Design review of the part built by this model. Coordinates are the model's own, in mm. Face numbers are marked on the shaded views. Round coordinates to 2 decimals unless told otherwise and drop trailing zeros. Loops run counter-clockwise (first coordinate to the right, second up) from the corner with the lowest first, then second, coordinate; pieces in that order, holes last. Notation, with made-up numbers: M -16,43 L 5,43 A7 cw 5,50 Z; hole C 8,79.5 d5. An arc over 180 degrees is marked long. Use a Markdown table: item, result.
from build123d import *

# Parameters (mm, degrees)
F0_W     = 19.05
F0_H     = 19.05
F1_DEPTH = 76.2
F3_DEPTH = 25.4
F5_D     = 6.5278
F5_DEPTH = 12.7
F5_TIP   = 1.9611489744
F7_D     = 3.7973
F7_DEPTH = 12.7
F7_TIP   = 1.1408240143
F8_SIZE2 = 0.762
F8_SIZE  = 0.762


with BuildPart() as f1:
    # F0 (on Right) → F1 (new body)
    with BuildSketch(Plane.YZ):
        with Locations((-9.525, 9.525)):
            Rectangle(F0_W, F0_H)
    extrude(amount=F1_DEPTH)

    # F2 (on face) → F3 (cut)
    with BuildSketch(Plane.XZ.offset(19.05)):
        Polygon((50.8027122421, 0), (38.1, 12.7027122421), (38.1, 0), align=None)
        Polygon((38.1, 0), (38.1, 12.7027122421), (25.3972877579, 0), align=None)
    extrude(amount=-F3_DEPTH, mode=Mode.SUBTRACT)

    # F5
    with Locations(Plane.XY.offset(19.05)):
        with Locations((15.875, -9.525), (60.325, -9.525)):
            Hole(F5_D / 2, depth=F5_DEPTH)
            with Locations((0, 0, -(F5_DEPTH + F5_TIP / 2))):  # 118° drill point
                Cone(0, F5_D / 2, F5_TIP, mode=Mode.SUBTRACT)

    # F7
    with Locations(Plane(origin=(0, 0, 0), x_dir=(1, 0, 0), z_dir=(0, 0, -1))):
        with Locations((6.35, 9.525), (69.85, 9.525)):
            Hole(F7_D / 2, depth=F7_DEPTH)
            with Locations((0, 0, -(F7_DEPTH + F7_TIP / 2))):  # 118° drill point
                Cone(0, F7_D / 2, F7_TIP, mode=Mode.SUBTRACT)

    # F8
    f8_edges = [f1.edges().sort_by_distance(p)[0] for p in [
        (76.2, -19.05, 9.525),
        (76.2, 0, 9.525),
        (0, -19.05, 9.525),
        (0, 0, 9.525),
    ]]
    chamfer(f8_edges, length=F8_SIZE, length2=F8_SIZE2)


solid = f1.part
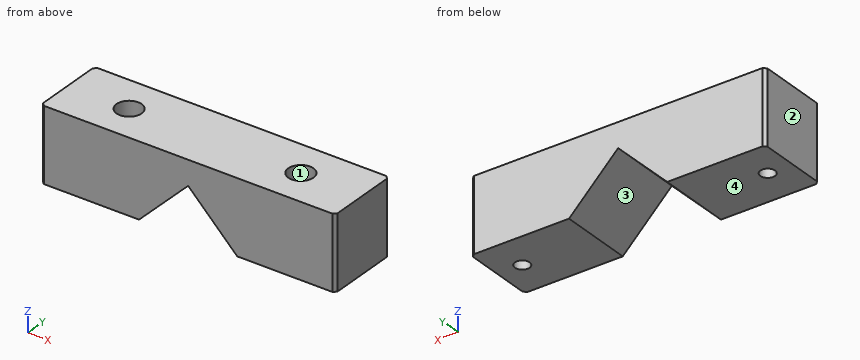
1. Wall thickness on line 1 along Y through (x, z) = (6.35, 6.75); line 2 along X through (y, z) = (-6.75, 12); line 3 along Y through (x, z) = (62, 11.25): over which ranges is each line inside the solid? List them lowest first. Write a range as from..to.
Check values:
| item | result |
|---|---|
| line 1 | y = -19.05..-11.42, -7.63..0 |
| line 2 | x = 0..14.16, 17.59..37.4, 38.8..58.61, 62.04..76.2 |
| line 3 | y = -19.05..-12.33, -6.72..0 |
2. Take a section at C-C on x = 41. Give the boundary of the cut face in (y, z).
Check values:
| item | result |
|---|---|
| outline | M -19.05,9.8 L 0,9.8 L 0,19.05 L -19.05,19.05 Z |
3. Insertion check: pin 1 (6 mm diameter, centred on x = 60.325, y = -9.525, fed in from +Z). The pin has a flat end and moves straight along its axis. Give the tip position at first contact, or say it passes through.
Check values:
| item | result |
|---|---|
| pin 1 | stops at z = 6.19 |
4. Take a section at A-A on y = -15.25. Give the boundary of the cut face in (x, z), and give its area (3 significant figures).
Check values:
| item | result |
|---|---|
| outline | M 0,0 L 25.4,0 L 38.1,12.7 L 50.8,0 L 76.2,0 L 76.2,19.05 L 0,19.05 Z |
| area | 1,290 mm² |
5. Take a section at B-B on z = 16.25. Give the boundary of the cut face in (x, y) (3 decimals).
Check values:
| item | result |
|---|---|
| outline | M 0,-18.288 L 0.762,-19.05 L 75.438,-19.05 L 76.2,-18.288 L 76.2,-0.762 L 75.438,0 L 0.762,0 L 0,-0.762 Z; hole C 15.875,-9.525 d6.528; hole C 60.325,-9.525 d6.528 |
6. The part is to be moulded in two halves that separate along X. For the marked faces 1, 2, 3 and 4, say which applies: pulls with the +X half, pulls with the -X half, needs draft (parallel to the pull), parting line crosses it, or undercut.
Check values:
| item | result |
|---|---|
| face 1 | undercut |
| face 2 | pulls with the -X half |
| face 3 | undercut |
| face 4 | needs draft |
